The listing builds one solid part. Answer for the finished solid, in the listing's coordinates (mm). A direction names the side the tool comes from. Give positions to 0.01 mm unless a question says otherwise; leave off trailing zeros. Loops run counter-clockwise (first coordinate to the right, second up) from the corner with the lowest first, then second, coordinate; pieces in that order, holes last. Notation, with made-up numbers: M 50,-30 L 80,-30 A19 ccw 80,-19 Z; hole C 53.25,7.25 d4. An arc over 180 degrees is marked long. One line per item, written item: value. Start each with the question number.
Q1. A cutting plane is placed at B-B, the plane y = 3.6. State how many separate pieces and enclosed holes the cut face has, and give its area (3 significant figures).
Q2. For faces 1 (the flat face through (43.267, 3, -88)), 2 (the flat face through (87, 3, 40.067)), 3 (the flat face through (-8, 3, 40.067)), determine the directions among +Z, -Z, +X, -X, +Y, -Y from which every point of the face is accessible in a straight line to the end or side of a thin tool.
Q3. A cutting plane is placed at A-A, the plane z = -21. Determine the outline of the cut face in (x, y), and give its area (3 significant figures).
Q4. The mould has two halves that part along Z. Classify faces 4 (the flat face through (-50, 3, -93)), 5 (the flat face through (-90, 3, -47)), 6 (the flat face through (21, 3, -96)): +Z half, -Z half, draft (parallel to the pull), parting line (faces both ways), or undercut.
Q5. Consider L1, parallel to X at y = 3.8, z = 0; L2, parallel to Z at x = -84.5, y = 2.7; L3, parallel to X at y = 3.25, z = -43.5. Determine where each line is inside the solid, lowest interval first.
Q6. Flat-ended cylindrical pins translate along their axes: pin 1 (1.6 mm diameter, centred on x = 84, y = 2.5, fed in from -Z); pin 2 (2.5 mm diameter, centred on y = 4.5, z = 0.5, fed in from +X); pin 3 (1.8 mm diameter, centred on x = 92.5, y = 3, fed in from +Z). Find the tip coordinate at first contact, or state that the pin passes through.
from build123d import *

# Parameters (mm, degrees)
SKETCH1_R           = 1.6
SKETCH1_W           = 6.2
SKETCH1_H           = 6.2
SKETCH1_W_2         = 80
SKETCH1_H_2         = 60
BOSS_EXTRUDE1_DEPTH = 6


with BuildPart() as part:
    # Sketch1 → Boss-Extrude1 (new body)
    with BuildSketch(Plane(origin=(0, 0, 0), x_dir=(1, 0, 0), z_dir=(0, 1, 0))):
        Polygon((85, 43.266666667), (90, 43.266666667), (90, 50), (96, 50), (96, 75), (90, 75), (90, 90), (75, 90), (75, 96), (50, 96), (50, 90), (43.266666667, 90), (43.266666667, 85), (44.566666667, 85), (44.566666667, 81.8), (43.266666667, 81.8), (43.266666667, 75), (40.066666667, 75), (40.066666667, 81.8), (38.766666667, 81.8), (38.766666667, 85), (40.066666667, 85), (40.066666667, 90), (33.333333333, 90), (33.333333333, 96), (8.333333333, 96), (8.333333333, 90), (1.6, 90), (1.6, 85), (2.9, 85), (2.9, 81.8), (1.6, 81.8), (1.6, 75), (-1.6, 75), (-1.6, 81.8), (-2.9, 81.8), (-2.9, 85), (-1.6, 85), (-1.6, 90), (-8.333333333, 90), (-8.333333333, 96), (-33.333333333, 96), (-33.333333333, 90), (-40.066666667, 90), (-40.066666667, 85), (-38.766666667, 85), (-38.766666667, 81.8), (-40.066666667, 81.8), (-40.066666667, 75), (-43.266666667, 75), (-43.266666667, 81.8), (-44.566666667, 81.8), (-44.566666667, 85), (-43.266666667, 85), (-43.266666667, 90), (-50, 90), (-50, 96), (-75, 96), (-75, 90), (-90, 90), (-90, 75), (-96, 75), (-96, 50), (-90, 50), (-90, 43.266666667), (-85, 43.266666667), (-85, 44.566666667), (-81.8, 44.566666667), (-81.8, 43.266666667), (-72, 43.266666667), (-72, 40.066666667), (-81.8, 40.066666667), (-81.8, 38.766666667), (-85, 38.766666667), (-85, 40.066666667), (-90, 40.066666667), (-90, 33.333333333), (-96, 33.333333333), (-96, 8.333333333), (-90, 8.333333333), (-90, 1.6), (-85, 1.6), (-85, 2.9), (-81.8, 2.9), (-81.8, 1.6), (-73.8, 1.6), (-73.8, -1.6), (-81.8, -1.6), (-81.8, -2.9), (-85, -2.9), (-85, -1.6), (-90, -1.6), (-90, -8.333333333), (-96, -8.333333333), (-96, -33.333333333), (-90, -33.333333333), (-90, -40.066666667), (-85, -40.066666667), (-85, -38.766666667), (-81.8, -38.766666667), (-81.8, -40.066666667), (-73.8, -40.066666667), (-73.8, -43.266666667), (-81.8, -43.266666667), (-81.8, -44.566666667), (-85, -44.566666667), (-85, -43.266666667), (-90, -43.266666667), (-90, -50), (-96, -50), (-96, -75), (-90, -75), (-90, -90), (90, -90), (90, -75), (96, -75), (96, -50), (90, -50), (90, -43.266666667), (85, -43.266666667), (85, -44.566666667), (81.8, -44.566666667), (81.8, -43.266666667), (73.8, -43.266666667), (73.8, -40.066666667), (81.8, -40.066666667), (81.8, -38.766666667), (85, -38.766666667), (85, -40.066666667), (90, -40.066666667), (90, -33.333333333), (96, -33.333333333), (96, -8.333333333), (90, -8.333333333), (90, -1.6), (85, -1.6), (85, -2.9), (81.8, -2.9), (81.8, -1.6), (73.8, -1.6), (73.8, 1.6), (81.8, 1.6), (81.8, 2.9), (85, 2.9), (85, 1.6), (90, 1.6), (90, 8.333333333), (96, 8.333333333), (96, 33.333333333), (90, 33.333333333), (90, 40.066666667), (85, 40.066666667), (85, 38.766666667), (81.8, 38.766666667), (81.8, 40.066666667), (72, 40.066666667), (72, 43.266666667), (81.8, 43.266666667), (81.8, 44.566666667), (85, 44.566666667), align=None)
        with Locations(Location((-26.6, -74.4, 0), (0, 0, 270))):
            Circle(SKETCH1_R, mode=Mode.SUBTRACT)
        with Locations((-62.7, -8.3)):
            Rectangle(SKETCH1_W, SKETCH1_H, mode=Mode.SUBTRACT)
        with Locations(Location((-62.7, 0, 0), (0, 0, 270))):
            Circle(SKETCH1_R, mode=Mode.SUBTRACT)
        with Locations((-8.3, -36.966666667)):
            Rectangle(SKETCH1_W, SKETCH1_H, mode=Mode.SUBTRACT)
        with Locations(Location((0, -36.966666667, 0), (0, 0, 270))):
            Circle(SKETCH1_R, mode=Mode.SUBTRACT)
        Rectangle(SKETCH1_W_2, SKETCH1_H_2, mode=Mode.SUBTRACT)
        with Locations(Location((26.6, -74.4, 0), (0, 0, 270))):
            Circle(SKETCH1_R, mode=Mode.SUBTRACT)
        with Locations((8.3, -36.966666667)):
            Rectangle(SKETCH1_W, SKETCH1_H, mode=Mode.SUBTRACT)
        with Locations((62.7, -8.3)):
            Rectangle(SKETCH1_W, SKETCH1_H, mode=Mode.SUBTRACT)
        with Locations(Location((62.7, 0, 0), (0, 0, 270))):
            Circle(SKETCH1_R, mode=Mode.SUBTRACT)
        with Locations((-62.7, 8.3)):
            Rectangle(SKETCH1_W, SKETCH1_H, mode=Mode.SUBTRACT)
        with Locations((-8.3, 36.966666667)):
            Rectangle(SKETCH1_W, SKETCH1_H, mode=Mode.SUBTRACT)
        with Locations(Location((0, 36.966666667, 0), (0, 0, 270))):
            Circle(SKETCH1_R, mode=Mode.SUBTRACT)
        with Locations((8.3, 36.966666667)):
            Rectangle(SKETCH1_W, SKETCH1_H, mode=Mode.SUBTRACT)
        with Locations((62.7, 8.3)):
            Rectangle(SKETCH1_W, SKETCH1_H, mode=Mode.SUBTRACT)
    extrude(amount=BOSS_EXTRUDE1_DEPTH)


solid = part.part
Answer block:
1. separate pieces: 1
1. enclosed holes: 15
1. area: 28,500 mm^2
2. face 1: -Z, +Y, -Y
2. face 2: +X, +Y, -Y
2. face 3: +Y, -Y
3. outline: M -96,0 L -40,0 L -40,6 L -96,6 Z; M 40,0 L 96,0 L 96,6 L 40,6 Z
3. area: 672 mm^2
4. face 4: draft
4. face 5: undercut
4. face 6: -Z half
5. L1: -73.8 to -64.3, -61.1 to -40, 40 to 61.1, 64.3 to 73.8
5. L2: -90 to -44.57, -38.77 to -2.9, 2.9 to 38.77, 44.57 to 90
5. L3: -90 to -85, -81.8 to 81.8, 85 to 90
6. pin 1: z = -90
6. pin 2: x = 90
6. pin 3: z = 75
